```python
from build123d import *

# Parameters (mm, degrees)
F0_R      = 18.677485
F0_R_2    = 6.197536
F1_DEPTH  = 47.752
F3_DEPTH  = 34.798
F4_R      = 24.770199
F4_R_2    = 12.651261
F5_DEPTH  = 1.27
F7_DEPTH  = 57.658
F9_DEPTH  = 57.404
F11_DEPTH = 57.658
F13_DEPTH = 57.15


with BuildPart() as f1:
    # F0 (on Top) → F1 (new body)
    with BuildSketch(Plane.XY):
        Circle(F0_R)
        Circle(F0_R_2, mode=Mode.SUBTRACT)
    extrude(amount=F1_DEPTH)

    # F2 (on Top) → F3 (join)
    with BuildSketch(Plane.XY):
        Polygon((23.808415, 41.237384), (-23.808415, 41.237384), (-47.61683, 0), (-23.808415, -41.237384), (23.808415, -41.237384), (47.61683, 0), align=None)
    extrude(amount=-F3_DEPTH)

    # F4 (on Top) → F5 (join)
    with BuildSketch(Plane.XY):
        Circle(F4_R)
        Circle(F4_R_2, mode=Mode.SUBTRACT)
    extrude(amount=F5_DEPTH)

    # F6 (on Top) → F7 (join)
    with BuildSketch(Plane.XY):
        Polygon((-12.180529, 35.239672), (-23.794444, 54.69878), (-34.839569, 34.911281), align=None)
    extrude(amount=F7_DEPTH)

    # F8 (on Top) → F9 (join)
    with BuildSketch(Plane.XY):
        Polygon((24.516974, 29.217048), (33.843096, 47.873281), (13.023263, 46.621824), align=None)
    extrude(amount=F9_DEPTH)

    # F10 (on Top) → F11 (join)
    with BuildSketch(Plane.XY):
        Polygon((-40.036782, -6.71368), (-45.977313, 10.143448), (-57.605748, -3.429767), align=None)
    extrude(amount=F11_DEPTH)

    # F12 (on Top) → F13 (join)
    with BuildSketch(Plane.XY):
        Polygon((54.162623, -6.586678), (51.286034, 8.247477), (39.877574, -1.660799), align=None)
    extrude(amount=F13_DEPTH)


solid = f1.part
```
Geometry: final body of the model. Coordinates: model frame, mm. A direction names the side the tool comes from. Coordinates: 2 decimals unless noted, no trailing zeros. Write each loop counter-clockwise with the first axis right and the second up, starting at its lowest first coordinate (ties: lowest second). Pieces come first, ordered by that corner, then holes. Notation, with made-up numbers: M -38.75,-5 L -6.75,-5 A8 ccw -6.75,10 Z; hole C 29,84.25 d3. An arc over 180 degrees is marked long. Answer as CSV lines item,"result". Start each with the question number.
Q1. Pin query (flat end, axial travel): P1, Ø9.5, axis at x = 22.5, y = 37.5, coming from the +Z side; P2, Ø5.5, axis at x = -25, y = 49.5, coming from the -Z side; P3, Ø1.5, axis at x = 27, z = -2, coming from the -Y side. Return the tip coordinate at first contact, or that it passes through.
Q2. Line query: line 1 (Y direction, x = 0, z = 34); line 2 (Y direction, x = 22.5, z = -16); line 3 (Z direction, x = 5, y = 24). Output: solid intervals per line, ascending. Write a range as from..to.
Q3. Reachability of faces 4 (the flat face through (0, -8, 47.752)), 5 (the flat face through (-35.546, 20.907, -17.155)), 6 (the flat face through (0, 41.237, -17)), 7 (the flat face through (-48.94, -5.05, 28.43)) from +Z, -Z, +X, -X, +Y, -Y: full face, straight path, thin tool, end or side. Return the list, or none.
Q4. Cut plane C-C on z = -14. Return the cut outline in (x, y).
Q5. Cut plane B-B on x = 0. Return the cut outline in (y, z), then the cut area to 3 significant figures.
Q6. Cut plane A-A on z = 15. Return the cut outline in (x, y).
Q7. Mould query, pull axis Y, two halves, no side actions, for faces 1 (the flat face through (23, 41, 57.404)), 2 (the cylindrical face through (-14.822, -11.365, 24.186)), 3 (the flat face through (-29.24, 44.94, 28.43)). Classes: released by +Y, released by -Y, zero draft, split by the parting line, or undercut.
Findings below:
1,P1,"stops at z = 57.4"
1,P2,"stops at z = 0"
1,P3,"stops at y = -37.01"
2,line 1,"y = -18.68..-6.2, 6.2..18.68"
2,line 2,"y = -41.24..41.24"
2,line 3,"z = -34.8..1.27"
3,face 4,"+Z, -Y"
3,face 5,"-Z, -X, +Y"
3,face 6,"-Z, +X, -X, +Y"
3,face 7,"+Z, -X, -Y"
4,outline,"M -47.62,0 L -23.81,-41.24 L 23.81,-41.24 L 47.62,0 L 23.81,41.24 L -23.81,41.24 Z"
5,outline,"M -41.24,-34.8 L 41.24,-34.8 L 41.24,0 L 24.77,0 L 24.77,1.27 L 18.68,1.27 L 18.68,47.75 L 6.2,47.75 L 6.2,0 L -6.2,0 L -6.2,47.75 L -18.68,47.75 L -18.68,1.27 L -24.77,1.27 L -24.77,0 L -41.24,0 Z"
5,area,"4,080 mm2"
6,outline,"M -57.61,-3.43 L -40.04,-6.71 L -45.98,10.14 Z; M -34.84,34.91 L -12.18,35.24 L -23.79,54.7 Z; C 0,0 d37.35; M 13.02,46.62 L 24.52,29.22 L 33.84,47.87 Z; M 39.88,-1.66 L 54.16,-6.59 L 51.29,8.25 Z; hole C 0,0 d12.4"
7,face 1,"zero draft"
7,face 2,"undercut"
7,face 3,"released by +Y"
